Here's the drawing with two shaded views (mm, measured from the low corner). I have some questions. A direction names the side the tool comes from. Give positions to 0.01 mm unless a question says otherwise; leave off trailing zeros. Loops run counter-clockwise (first coordinate to the right, second up) from the corner with the lowest first, then second, coordinate; pieces in that order, holes last. Notation, with made-up numbers: M 26.5,32 L 81.5,32 A22 cw 81.5,58 Z; hole C -13.75,65.25 d8. An arc over 180 degrees is marked long. Use a Markdown table: item, result. Add a question column.
1) Which directions (+Z, -Z, +X, -X, +Y, -Y) give clear straight access to the entire face, cutting with the end or side of a thin tool? Please do the marked faces 1 and 2.
2) Suppose I cut it at B-B on y = 12.5. List the corners of the cut face in (x, z) for me.
3) Suppose I cut it at C-C on z = 29. List the corners of the cut face in (x, y) for me, and give its area (3 significant figures).
4) Suppose I cut it at A-A on x = 12.5. List the corners of the cut face in (y, z) for me.
5) If I drill on line 1 along Z through (x, y) = (9, 5.25); line 2 along Y through (x, z) = (21.5, 28.9); line 3 along Z through (x, y) = (11.75, 16.5), over which ranges is the centre line in solid material (lowest first)? Write a range as [from, to].
6) Suppose I cut it at D-D on z = 23. List the corners of the cut face in (x, y) for me.
7) Will these pins go through, and if not, where does the flat tip stop? pin 1 Ø5 at (y, z) = (18.5, 22.5) entering from -X; pin 2 Ø8 at (x, z) = (6.5, 33.5) entering from +Y; pin 3 Ø4 at (x, z) = (9, 9) entering from -Y.
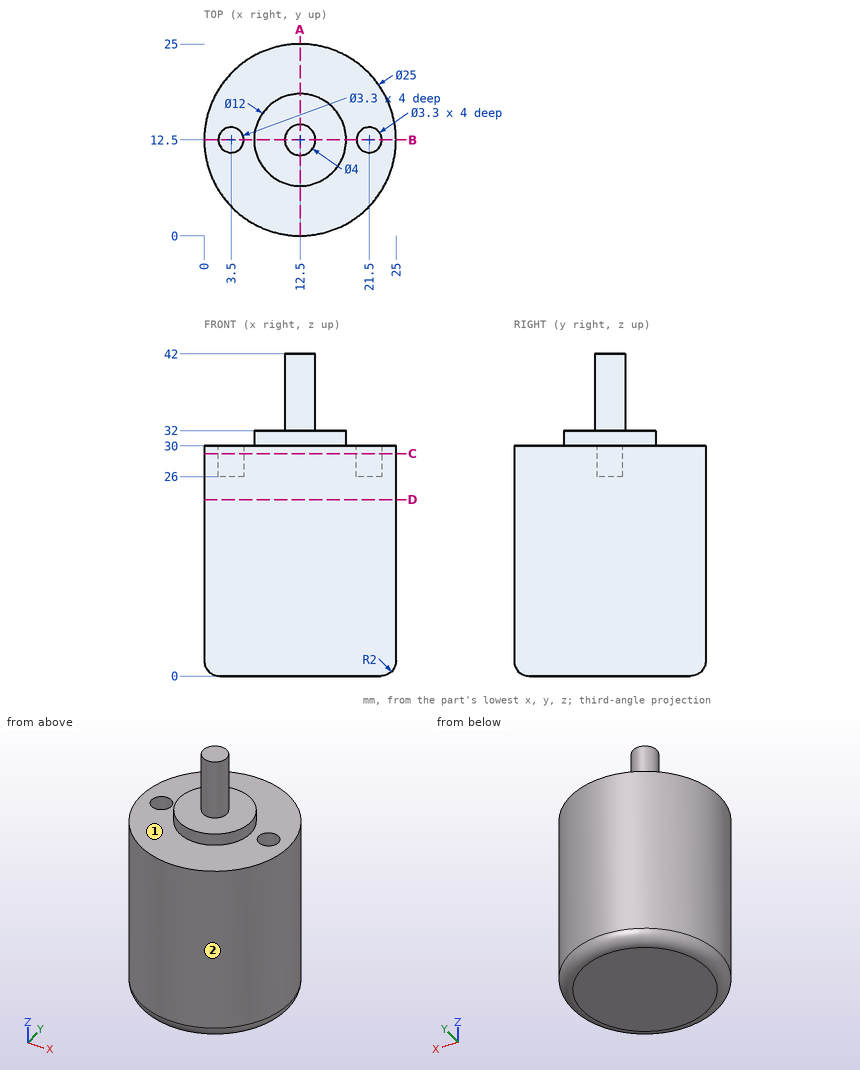
Answer block:
| question | item | result |
|---|---|---|
| 1 | face 1 | +Z |
| 1 | face 2 | +Z, -Z |
| 2 | outline | M 0,2 A2 ccw 2,0 L 23,0 A2 ccw 25,2 L 25,30 L 23.15,30 L 23.15,26 L 19.85,26 L 19.85,30 L 18.5,30 L 18.5,32 L 14.5,32 L 14.5,42 L 10.5,42 L 10.5,32 L 6.5,32 L 6.5,30 L 5.15,30 L 5.15,26 L 1.85,26 L 1.85,30 L 0,30 Z |
| 3 | outline | C 12.5,12.5 d25; hole C 3.5,12.5 d3.3; hole C 21.5,12.5 d3.3 |
| 3 | area | 474 mm^2 |
| 4 | outline | M 0,2 A2 ccw 2,0 L 23,0 A2 ccw 25,2 L 25,30 L 18.5,30 L 18.5,32 L 14.5,32 L 14.5,42 L 10.5,42 L 10.5,32 L 6.5,32 L 6.5,30 L 0,30 Z |
| 5 | line 1 | z = [0, 30] |
| 5 | line 2 | y = [3.83, 10.85], [14.15, 21.17] |
| 5 | line 3 | z = [0, 32] |
| 6 | outline | C 12.5,12.5 d25 |
| 7 | pin 1 | stops at x = 0.5 |
| 7 | pin 2 | stops at y = 24.32 |
| 7 | pin 3 | stops at y = 0.09 |
